Read the model definition and answer for the solid it produces. Units are mm, in the model's axes. A direction names the side the tool comes from. Coordinates: 2 decimals unless noted, no trailing zeros. Loops run counter-clockwise (first coordinate to the right, second up) from the corner with the lowest first, then second, coordinate; pieces in that order, holes last. Notation, with made-up numbers: M -38.75,22 L -25.75,22 A7 ccw -25.75,26 Z; hole C 9,51 d7. An arc over 180 degrees is marked long. Put each result on its own line as item: value.
from build123d import *

# Parameters (mm, degrees)
F1_R     = 7.5
F2_DEPTH = 10
F3_START = 10
F3_DEPTH = 5
F4_SIZE  = 1
F6_DEPTH = 6
F7_SIZE  = 0.5


with BuildPart() as f2:
    # F1 (on Top) → F2 (new body)
    with BuildSketch(Plane.XY):
        Circle(F1_R)
    extrude(amount=F2_DEPTH)

    # F0 (on Top) → F3 (join)
    with BuildSketch(Plane.XY.offset(F3_START)):
        with BuildLine():
            Line((3.3952172243, 3.25), (-3.3952172243, 3.25))
            ThreePointArc((-3.3952172243, 3.25), (-4.7, 0), (-3.3952172243, -3.25))
            Line((-3.3952172243, -3.25), (3.3952172243, -3.25))
            ThreePointArc((3.3952172243, -3.25), (4.7, 0), (3.3952172243, 3.25))
        make_face()
    extrude(amount=F3_DEPTH)

    # F4
    f4_edges = [f2.edges().sort_by_distance(p)[0] for p in [
        (-4.7, 0, 15),
        (0, -3.25, 15),
        (4.7, 0, 15),
        (0, 3.25, 15),
    ]]
    chamfer(f4_edges, length=F4_SIZE)

    # F5 (on face) → F6 (cut)
    with BuildSketch(Plane(origin=(0, 0, 0), x_dir=(1, 0, 0), z_dir=(0, 0, -1))):
        with BuildLine():
            Line((-2.2118996361, -2.1), (2.2118996361, -2.1))
            ThreePointArc((2.2118996361, -2.1), (3.05, 0), (2.2118996361, 2.1))
            Line((2.2118996361, 2.1), (-2.2118996361, 2.1))
            ThreePointArc((-2.2118996361, 2.1), (-3.05, 0), (-2.2118996361, -2.1))
        make_face()
    extrude(amount=-F6_DEPTH, mode=Mode.SUBTRACT)

    # F7
    f7_edges = [f2.edges().sort_by_distance(p)[0] for p in [
        (-7.5, 0, 0),
        (0, -2.1, 0),
        (3.05, 0, 0),
        (0, 2.1, 0),
        (-3.05, 0, 0),
    ]]
    chamfer(f7_edges, length=F7_SIZE)


solid = f2.part
1) Find section C-C, the plane z = 2.75. Write down the section's boundary in (x, y), plus the area to 3 significant figures.
Answer list:
outline: C 0,0 d15; hole M -2.21,-2.1 L 2.21,-2.1 A3.05 ccw 2.21,2.1 L -2.21,2.1 A3.05 ccw Z
area: 153 mm^2
2) Straight lines are drawn through the part: line 1 (Y direction, x = -2, z = 4.5); line 2 (Z direction, x = -4.25, y = 5); line 3 (Y direction, x = 0.25, z = 13). For each, find the intervals that lie inside material, in ascending order. Write a range as [from, to].
Answer list:
line 1: y = [-7.23, -2.1], [2.1, 7.23]
line 2: z = [0, 10]
line 3: y = [-3.25, 3.25]
3) Determine the mould class of faces 1 (the flat face through (0.05, 2.74, 14.51)), 2 (the conical face through (-3.19, -0.04, 0.36)), 3 (the flat face through (0, 0, 6)), 4 (the conical face through (4.1, 0, 14.6)) for opening direction Y: released by +Y, released by -Y, zero draft, split by the parting line, or undercut.
Answer list:
face 1: released by +Y
face 2: undercut
face 3: undercut
face 4: split by the parting line
4) Which of the six approach directions +Z, -Z, +X, -X, +Y, -Y give full straight-line access (tool end or side, diameter ignored) to faces 5 (the cylindrical face through (3.05, 0.03, 3.21)), 6 (the cylindrical face through (-4.7, 0.1, 12)), 7 (the flat face through (0, 3.25, 12)), 8 (the flat face through (0, -3.25, 12))?
Answer list:
face 5: -Z
face 6: +Z, -X
face 7: +Z, +X, -X, +Y
face 8: +Z, +X, -X, -Y
5) Find section B-B, the plane y = 0. Write down the section's boundary in (x, z).
Answer list:
outline: M -7.5,0.5 L -7,0 L -3.55,0 L -3.05,0.5 L -3.05,6 L 3.05,6 L 3.05,0.5 L 3.55,0 L 7,0 L 7.5,0.5 L 7.5,10 L 4.7,10 L 4.7,14 L 3.7,15 L -3.7,15 L -4.7,14 L -4.7,10 L -7.5,10 Z
6) Find section A-A, the plane x = 0. Write down the section's boundary in (y, z).
Answer list:
outline: M -7.5,0.5 L -7,0 L -2.6,0 L -2.1,0.5 L -2.1,6 L 2.1,6 L 2.1,0.5 L 2.6,0 L 7,0 L 7.5,0.5 L 7.5,10 L 3.25,10 L 3.25,14 L 2.25,15 L -2.25,15 L -3.25,14 L -3.25,10 L -7.5,10 Z
7) Given pin 1 Ø2 at (y, z) = (5.5, 9.5) entering from +X; pin 2 Ø2 at (x, z) = (-3, 5) entering from -Y; pin 3 Ø4.5 at (x, z) = (0.5, 12.5) entering from +Y, each flat-ended and moving along its own axis, determine where each tip first touches the part or whether it passes through.
Answer list:
pin 1: stops at x = 6
pin 2: stops at y = -7.23
pin 3: stops at y = 3.25
